from build123d import *

# Parameters (mm, degrees)
EXTRUDE_1_DEPTH     = 4
SKETCH_5_R          = 0.9
CUT_EXTRUDE_1_DEPTH = 10


with BuildPart() as part:
    # 草图1 → 凸台-拉伸1 (new body)
    with BuildSketch(Plane(origin=(0, 0, 0), x_dir=(1, 0, 0), z_dir=(0, 1, 0))):
        with BuildLine():
            Line((3.5, 7.5), (3.5, -7.5))
            Line((3.5, -7.5), (-3.5, -7.5))
            Line((-3.5, -7.5), (-3.5, 7.5))
            Line((-3.5, 7.5), (-12.209915195, 15.754536771))
            ThreePointArc((-12.209915195, 15.754536771), (-39.438437854, 86.09778223), (-2.187829675, 151.687086375))
            Line((-2.187829675, 151.687086375), (-2.187829675, 147.687086375))
            ThreePointArc((-2.187829675, 147.687086375), (-32.965427594, 82.391199834), (-5.209915195, 15.754536771))
            Line((-5.209915195, 15.754536771), (3.5, 7.5))
        make_face()
    extrude(amount=EXTRUDE_1_DEPTH)

    # 草图5 → 切除-拉伸1 (cut)
    with BuildSketch(Plane(origin=(0, 4, 0), x_dir=(1, 0, 0), z_dir=(0, 1, 0))):
        with Locations(Location((0, -3.5, 0), (0, 0, 270))):
            Circle(SKETCH_5_R)
        with Locations(Location((0, 2.5, 0), (0, 0, 270))):
            Circle(SKETCH_5_R)
    extrude(amount=-CUT_EXTRUDE_1_DEPTH, mode=Mode.SUBTRACT)


solid = part.part
CAD build for the part. Positions are in the model's coordinates, mm. A direction names the side the tool comes from. Coordinates: 2 decimals unless noted, no trailing zeros. Loops run counter-clockwise (first coordinate to the right, second up) from the corner with the lowest first, then second, coordinate; pieces in that order, holes last. Notation, with made-up numbers: (-5.75, -33.75) - (-1.75, -33.75) arc R10 cw to (-1.75, -23.75) - close; hole circle Ø8 at (71.5, 24.25). An arc over 180 degrees is marked (long way). Use one line per item in the form item = value. Start each with the question number.
1) Band-saw the part on A-A (x = -14). Give the cut face in (y, z), and give its area (3 significant figures).
2) Flat gauge pins, fed straight in: pin 1 (2 mm diameter, centred on x = -9, y = 2.5, fed in from +Z); pin 2 (3 mm diameter, centred on x = 0, z = 3.5, fed in from -Y); pin 3 (1 mm diameter, centred on x = -5.5, y = 3.5, fed in from -Z). Where does each tip first touch, or does it go through?
3) Band-saw the part on D-D (z = -114.5). Give the cut face in (x, y).
4) Tool access for faces 1 (the face through (-3.5, 2, 0)), 2 (the face through (-0.92, 1.97, -11.69)), 3 (the face through (-34, 0, -72)): list every direction of +Z, -Z, +X, -X, +Y, -Y with a clear straight run to the whole face (end or side of a thin tool).
5) Band-saw the part on B-B (y = 1.5). Give the cut face in (x, z).
6) Two-plate mould, pull along Z, no slides. Class faces 4 (the face through (-2.188, 2, -150)), 5 (the face through (-32.936, 1.972, -83.431)), 6 (the face through (0, 2, 7.5)): +Z half, -Z half, draft (parallel to the pull), parting line (faces both ways), or undercut.
7) Drill centre lines: L1, parallel to X at y = 2.8, z = 3.5; L2, parallel to Z at x = -20, y = 0.25; L3, parallel to Z at x = -16.5, y = 0.5. Where is each one in solid material? Low to high. Write a range as from..to.
8) Band-saw the part on C-C (z = -5.5). Give the cut face in (x, y), and give its area (3 significant figures).
Check values:
q1.outline = (0, -141.75) - (4, -141.75) - (4, -135.3) - (0, -135.3) - close; (0, -25.4) - (4, -25.4) - (4, -17.5) - (0, -17.5) - close
q1.area = 57.4 mm2
q2.pin_1 = -11.76
q2.pin_2 = 0
q2.pin_3 = -149.63
q3.outline = (-32.47, 0) - (-26.18, 0) - (-26.18, 4) - (-32.47, 4) - close
q4.face_1 = +Z, -X, +Y, -Y
q4.face_2 = +X, +Y, -Y
q4.face_3 = +Z, -Z, +X, -X, -Y
q5.outline = (-12.21, -15.75) arc R88 ccw to (-2.19, -151.69) - (-2.19, -147.69) arc R89 cw to (-5.21, -15.75) - (3.5, -7.5) - (3.5, 7.5) - (-3.5, 7.5) - (-3.5, -7.5) - close; hole circle Ø1.8 at (0, -2.5); hole circle Ø1.8 at (0, 3.5)
q6.face_4 = draft
q6.face_5 = undercut
q6.face_6 = +Z half
q7.L1 = -3.5..-0.9, 0.9..3.5
q7.L2 = -135.09..-126.65, -34.06..-24.17
q7.L3 = -139.14..-131.96, -28.75..-20.11
q8.outline = (-3.5, 0) - (3.5, 0) - (3.5, 4) - (-3.5, 4) - close
q8.area = 28.0 mm2
